Read the model definition and answer for the solid it produces. Units are mm, in the model's axes. Give positions to 0.01 mm unless a question says otherwise; leave off trailing zeros. Loops run counter-clockwise (first coordinate to the right, second up) from the corner with the lowest first, then second, coordinate; pieces in that order, holes last. Notation, with made-up numbers: (55.25, -24) - (112.25, -24) arc R26 ccw to (112.25, 8) - close; hole circle Ø2 at (-38, 38). An arc over 180 degrees is marked (long way). Put each result on its own line as item: value. Start each with the question number.
1. For a pull along X with two mould halves and no side action, classify faces 1 (the cylindrical face through (12.932, 5.362, 7.409)), 2 (the flat face through (4, 15, 15)), 3 (the cylindrical face through (22.4, -7.1, 7.4)) as released by +X, released by -X, zero draft, split by the parting line, or undercut.
2. Consider L1, parallel to Y at x = 0, z = 10.5; L2, parallel to X at y = -9, z = 1; L3, parallel to Y at x = -5, z = 8.5. Determine where each line is inside the solid, lowest interval first. Write a range as from..to.
3. A cutting plane is placed at A-A, the plane y = 0. Determine the outline of the cut face in (x, z).
4. A cutting plane is placed at C-C, the plane z = 11. Determine the outline of the cut face in (x, y).
5. Given pin 1 Ø17 at (x, y) = (0, 0) entering from +Z; pin 2 Ø1 at (y, z) = (18, 13.5) entering from -X; pin 3 Ø1 at (y, z) = (-7, 12) entering from +X; pin 4 Ø1.5 at (y, z) = (-15.5, 4) entering from -X, each flat-ended and moving along its own axis, determine where each tip first touches the part or whether it passes through.
Autodesk Inventor part; units mm, degrees
ref_plane "YZ Plane" through (0, 0, 0) normal (1, 0, 0) x (0, 1, 0)
ref_plane "XZ Plane" through (0, 0, 0) normal (0, 1, 0) x (-1, 0, 0)
ref_plane "XY Plane" through (0, 0, 0) normal (0, 0, 1) x (1, 0, 0)
sketch "Sketch1" plane through (0, 0, 0) normal (0, 0, 1) x (1, 0, 0)
  circle A0 centre (0, 0) radius 14
  circle A1 centre (0, 0) radius 23.5
  dimension "d0" = 28
  dimension "d1" = 47
extrude "Extrusion1" add sketch "Sketch1" along normal blind 15
fillet "Fillet1" radius 2 2 edges at (-23.5, 0, 15) (-23.5, 0, 0)
fillet "Fillet2" radius 1 2 edges at (-14, 0, 0) (-14, 0, 15)
properties part number "U51105" material "Steel, Carbon"
Return value:
1. face 1: undercut
1. face 2: zero draft
1. face 3: split by the parting line
2. L1: y = -23.5..-14, 14..23.5
2. L2: x = -21.42..-10.72, 10.72..21.42
2. L3: y = -22.96..-13.08, 13.08..22.96
3. outline: (-23.5, 2) arc R2 ccw to (-21.5, 0) - (-15, 0) arc R1 ccw to (-14, 1) - (-14, 14) arc R1 ccw to (-15, 15) - (-21.5, 15) arc R2 ccw to (-23.5, 13) - close; (14, 1) arc R1 ccw to (15, 0) - (21.5, 0) arc R2 ccw to (23.5, 2) - (23.5, 13) arc R2 ccw to (21.5, 15) - (15, 15) arc R1 ccw to (14, 14) - close
4. outline: circle Ø47 at (0, 0); hole circle Ø28 at (0, 0)
5. pin 1: passes through
5. pin 2: stops at x = -15.61
5. pin 3: stops at x = 22.58
5. pin 4: stops at x = -18.29
